Could you check a few things on this model? Use its own coordinates, in mm. A direction names the side the tool comes from. Give positions to 0.01 mm unless a question says otherwise; leave off trailing zeros. Order: outer loops, then holes, each group sorted by start corner. A loop starts at its lowest first (then second) coordinate and runs counter-clockwise, first axis right, second up. Notation, with made-up numbers: M -14.5,85.25 L 9.5,85.25 A24 cw 9.5,102.25 Z; hole C 5,46.25 d9. An arc over 180 degrees is marked long. Return JSON: item names as keys, results as strings. Group by question number.
```python
from build123d import *

# Parameters (mm, degrees)
SKETCH1_W               = 210
SKETCH1_H               = 61.270358306
BOSS_EXTRUDE1_DEPTH     = 4
SKETCH2_R               = 1.5
CUT_EXTRUDE1_DEPTH      = 5
SKETCH3_R               = 2
CUT_EXTRUDE2_DEPTH      = 5
CUT_EXTRUDE3_DEPTH      = 5
MIRROR3_COPY_1_SKETCH_R = 2
MIRROR3_COPY_1_DEPTH    = 5
MIRROR3_COPY_2_DEPTH    = 5


with BuildPart() as part:
    # Sketch1 → Boss-Extrude1 (new body)
    with BuildSketch(Plane(origin=(0, 0, 0), x_dir=(0, 0, -1), z_dir=(1, 0, 0))):
        Rectangle(SKETCH1_W, SKETCH1_H)
    extrude(amount=BOSS_EXTRUDE1_DEPTH)

    # Sketch2 → Cut-Extrude1 (cut, through all)
    with BuildSketch(Plane(origin=(4, 0, 0), x_dir=(0, 0, -1), z_dir=(1, 0, 0))):
        with Locations((-90, 0)):
            Circle(SKETCH2_R)
    cut_extrude1 = extrude(amount=-CUT_EXTRUDE1_DEPTH, mode=Mode.SUBTRACT)

    # Sketch3 → Cut-Extrude2 (cut, through all)
    with BuildSketch(Plane(origin=(4, 0, 0), x_dir=(0, 0, -1), z_dir=(1, 0, 0))):
        with Locations((-17.7, 17.5)):
            Circle(SKETCH3_R)
    cut_extrude2 = extrude(amount=-CUT_EXTRUDE2_DEPTH, mode=Mode.SUBTRACT)

    # Sketch4 → Cut-Extrude3 (cut, through all)
    with BuildSketch(Plane(origin=(4, 0, 0), x_dir=(0, 0, -1), z_dir=(1, 0, 0))):
        with BuildLine():
            Line((-89, 10), (-35.2, 10))
            ThreePointArc((-35.2, 10), (-29.896699141, 12.196699141), (-27.7, 17.5))
            ThreePointArc((-27.7, 17.5), (-24.771067812, 24.571067812), (-17.7, 27.5))
            Line((-17.7, 27.5), (0, 27.5))
            Line((0, 27.5), (0, 30.635179153))
            Line((0, 30.635179153), (-105, 30.635179153))
            Line((-105, 30.635179153), (-105, 0))
            ThreePointArc((-105, 0), (-98.433981132, 7.294369811), (-89, 10))
        make_face()
    cut_extrude3 = extrude(amount=-CUT_EXTRUDE3_DEPTH, mode=Mode.SUBTRACT)

    # Mirror2: Cut-Extrude2, Cut-Extrude3 across plane
    add(cut_extrude2.mirror(Plane.ZX), mode=Mode.SUBTRACT)
    add(cut_extrude3.mirror(Plane.ZX), mode=Mode.SUBTRACT)

    # Mirror3: Cut-Extrude3, Cut-Extrude1, Cut-Extrude2 across plane
    add(cut_extrude3.mirror(Plane.XY), mode=Mode.SUBTRACT)
    add(cut_extrude1.mirror(Plane.XY), mode=Mode.SUBTRACT)
    add(cut_extrude2.mirror(Plane.XY), mode=Mode.SUBTRACT)

    # Mirror3 copy 1 sketch → Mirror3 copy 1 (cut, through all)
    with BuildSketch(Plane(origin=(4, 0, 0), x_dir=(0, 0, 1), z_dir=(1, 0, 0))):
        with Locations((-17.7, 17.5)):
            Circle(MIRROR3_COPY_1_SKETCH_R)
    extrude(amount=-MIRROR3_COPY_1_DEPTH, mode=Mode.SUBTRACT)

    # Mirror3 copy 2 sketch → Mirror3 copy 2 (cut, through all)
    with BuildSketch(Plane(origin=(4, 0, 0), x_dir=(0, 0, 1), z_dir=(1, 0, 0))):
        with BuildLine():
            Line((-89, 10), (-35.2, 10))
            ThreePointArc((-35.2, 10), (-29.896699141, 12.196699141), (-27.7, 17.5))
            ThreePointArc((-27.7, 17.5), (-24.771067812, 24.571067812), (-17.7, 27.5))
            Line((-17.7, 27.5), (0, 27.5))
            Line((0, 27.5), (0, 30.635179153))
            Line((0, 30.635179153), (-105, 30.635179153))
            Line((-105, 30.635179153), (-105, 0))
            ThreePointArc((-105, 0), (-98.433981132, 7.294369811), (-89, 10))
        make_face()
    extrude(amount=-MIRROR3_COPY_2_DEPTH, mode=Mode.SUBTRACT)


solid = part.part
```
1. I need wall thicknesses on L1, parallel to Y at x = 1.2, z = -17.7; L2, parallel to Z at x = 0.95, y = -17.5; L3, parallel to Y at x = 2.45, z = 90. Which ranges of each line are inside material? Lowest first, please. Write a range as from..to.
2. If we mould it in two halves opening along Y, with no side actions, what happens to faces 1 (the cylindrical face through (2.03, -24.49, -24.85)), 2 (the flat face through (2, 27.5, 0)), 3 (the cylindrical face through (2.028, -18.852, -19.174))? For each: pulls with the +Y half, pulls with the -Y half, needs draft (parallel to the pull), parting line crosses it, or undercut.
3. Imagine slicing it at B-B, the plane y = -13. Please give me the cut outline in (x, z), plus the area to 3 significant figures.
4. Imagine slicing it at A-A, the plane x = 2.5. Please give me the cut outline in (y, z), plus the area to 3 significant figures.
5. For pin 1 (2 mm diameter, centred on x = 1.5, z = -51.5, fed in from +Y); pin 2 (1.2 mm diameter, centred on x = 2.5, z = 71.5, fed in from -Y); pin 3 (1.5 mm diameter, centred on x = 1, y = 16, fed in from +Z), each with a flat end and sliding along its axis, tell me the tip position at first contact or that it passes through.
6. Imagine slicing it at C-C, the plane z = -67. Please give me the cut outline in (x, y).
7. Which directions (+Z, -Z, +X, -X, +Y, -Y) give clear straight access to the entire face, cutting with the end or side of a thin tool? Please do faces 4 (the flat face through (2, 10, 62)), 5 (the flat face through (2, -10, -62)), 6 (the flat face through (2, 10, -62)), 7 (the flat face through (2, -10, 62)), 8 (the cylindrical face through (2.028, 18.852, 19.174)).
Values:
{
 "1": {"L1": "y = -27.5..-19.5, -15.5..15.5, 19.5..27.5", "L2": "z = -27.7..-19.7, -15.7..15.7, 19.7..27.7", "L3": "y = -9.97..-1.5, 1.5..9.97"},
 "2": {"face 1": "pulls with the -Y half", "face 2": "pulls with the +Y half", "face 3": "undercut"},
 "3": {"outline": "M 0,-29.2 L 4,-29.2 L 4,29.2 L 0,29.2 Z", "area": "234 mm²"},
 "4": {"outline": "M -27.5,-17.7 A10 ccw -17.5,-27.7 A7.5 cw -10,-35.2 L -10,-89 A17.8 ccw 0,-105 A17.8 ccw 10,-89 L 10,-35.2 A7.5 cw 17.5,-27.7 A10 ccw 27.5,-17.7 L 27.5,17.7 A10 ccw 17.5,27.7 A7.5 cw 10,35.2 L 10,89 A17.8 ccw 0,105 A17.8 ccw -10,89 L -10,35.2 A7.5 cw -17.5,27.7 A10 ccw -27.5,17.7 Z; hole C -17.5,-17.7 d4; hole C -17.5,17.7 d4; hole C 0,-90 d3; hole C 0,90 d3; hole C 17.5,-17.7 d4; hole C 17.5,17.7 d4", "area": "5,860 mm²"},
 "5": {"pin 1": "stops at y = 10", "pin 2": "stops at y = -10", "pin 3": "stops at z = 28.05"},
 "6": {"outline": "M 0,-10 L 4,-10 L 4,10 L 0,10 Z"},
 "7": {"face 4": "+Z, +X, -X, +Y", "face 5": "-Z, +X, -X, -Y", "face 6": "-Z, +X, -X, +Y", "face 7": "+Z, +X, -X, -Y", "face 8": "+X, -X"}
}
